from build123d import *

# Parameters (mm, degrees)
SKETCH_1_R               = 2.9
EXTRUDE_1_DEPTH          = 35
SKETCH_2_W               = 0.4
SKETCH_2_H               = 5.450532248
CUT_EXTRUDE_1_DEPTH      = 12
CUT_EXTRUDE_2_DEPTH      = 10
CUT_EXTRUDE_2_DEPTH_BACK = 10
SKETCH_3_R               = 1


with BuildPart() as part:
    # 草图1 → 凸台-拉伸1 (new body)
    with BuildSketch(Plane(origin=(0, 0, 0), x_dir=(0, 0, -1), z_dir=(1, 0, 0))):
        Circle(SKETCH_1_R)
    extrude(amount=EXTRUDE_1_DEPTH)

    # 草图2 → 切除-拉伸1 (cut)
    with BuildSketch(Plane.ZY):
        with Locations((0, 0.396255312)):
            Rectangle(SKETCH_2_W, SKETCH_2_H)
    extrude(amount=-CUT_EXTRUDE_1_DEPTH, mode=Mode.SUBTRACT)

    # 草图3 → 切除-拉伸2 (cut, two sides: drawn at the far end of the back side and taken through both)
    with BuildSketch(Plane(origin=(0, 0, 0.2), x_dir=(-1, 0, 0), z_dir=(0, 0, -1)).offset(-CUT_EXTRUDE_2_DEPTH_BACK)):
        with Locations(Location((-3, -0.003452386, 0), (0, 0, 270))):
            Circle(SKETCH_3_R)
        with Locations(Location((-30, -0.003452386, 0), (0, 0, 270))):
            Circle(SKETCH_3_R)
    extrude(amount=CUT_EXTRUDE_2_DEPTH + CUT_EXTRUDE_2_DEPTH_BACK, mode=Mode.SUBTRACT)


solid = part.part
Input: part model. Units: mm. Frame: model coordinates. A direction names the side the tool comes from. Round coordinates to 2 decimals unless told otherwise and drop trailing zeros. Loops run counter-clockwise (first coordinate to the right, second up) from the corner with the lowest first, then second, coordinate; pieces in that order, holes last. Notation, with made-up numbers: (-21, 34) -> (-11, 34) arc R25 ccw to (-11, 67) -> close; hole circle Ø5 at (-3.75, -7.5). An arc over 180 degrees is marked (long way). Answer as a JSON object with one key per item and string values. Group by question number.
1) Section query A-A on x = 3. Output: boundary loops of the cut face in (y, z), plus the area to 3 significant figures.
2) Draft query along X for faces 3 (the flat face through (35, 0, 0)), 4 (the flat face through (6, 0, 0.2)), 5 (the cylindrical face through (29, 0, 0)). Return one class per face: +X half, -X half, draft (parallel to the pull), parting line (faces both ways), or undercut.
3) Section query B-B on z = 2.35. Output: boundary loops of the cut face in (x, y), plus the area to 3 significant figures.
4) Ray query, L1, parallel to X at y = -0.5, z = 2.3; L2, parallel to X at y = 0.6, z = -0.25; L3, parallel to Y at x = 3, z = 2.05. Return the intervals inside material, ascending.
5) Pin query (flat end, axial travel): pin 1 (2 mm diameter, centred on x = 8, z = -2.5, fed in from -Y); pin 2 (1.8 mm diameter, centred on x = 30, y = 0, fed in from +Z); pin 3 (3 mm diameter, centred on x = 16.5, y = -2, fed in from -Z). Return the tip coordinate at first contact, or that it passes through.
6) Section query C-C on y = 1.45. Output: boundary loops of the cut face in (x, z).
7) Reachability of faces 1 (the flat face through (6, 0, -0.2)), 2 (the cylindrical face through (3.38, -0.93, -1.53)) from +Z, -Z, +X, -X, +Y, -Y: full face, straight path, thin tool, end or side. Return the list, or none.
8) Section query D-D on x = 30. Output: boundary loops of the cut face in (y, z).
Reply:
{
 "1": {"outline": "(-2.33, -0.2) -> (-2.33, 0.2) -> (-1, 0.2) -> (-1, 2.72) arc R2.9 ccw to (-1, -2.72) -> (-1, -0.2) -> close; (1, -2.72) arc R2.9 ccw to (2.89, -0.2) -> (1, -0.2) -> close; (1, 0.2) -> (2.89, 0.2) arc R2.9 ccw to (1, 2.72) -> close", "area": "13.8 mm2"},
 "2": {"face 3": "+X half", "face 4": "draft", "face 5": "undercut"},
 "3": {"outline": "(0, -1.7) -> (35, -1.7) -> (35, 1.7) -> (0, 1.7) -> close; hole circle Ø2 at (3, 0); hole circle Ø2 at (30, 0)", "area": "113 mm2"},
 "4": {"L1": "x = 0 to 2.13, 3.87 to 29.13, 30.87 to 35", "L2": "x = 0 to 2.2, 3.8 to 29.2, 30.8 to 35", "L3": "y = -2.05 to -1, 1 to 2.05"},
 "5": {"pin 1": "stops at y = -2.48", "pin 2": "passes through", "pin 3": "stops at z = -2.86"},
 "6": {"outline": "(0, -2.51) -> (35, -2.51) -> (35, 2.51) -> (0, 2.51) -> (0, 0.2) -> (12, 0.2) -> (12, -0.2) -> (0, -0.2) -> close"},
 "7": {"face 1": "-X, +Y", "face 2": "+Z, -Z"},
 "8": {"outline": "(-1, -2.72) -> (-1, 2.72) arc R2.9 ccw to start; (1, -2.72) arc R2.9 ccw to (1, 2.72) -> close"}
}
